Here's how the part is built. I have some questions about the finished solid (model axes, mm). Coordinates: 2 decimals unless noted, no trailing zeros. Loops run counter-clockwise (first coordinate to the right, second up) from the corner with the lowest first, then second, coordinate; pieces in that order, holes last. Notation, with made-up numbers: (-40, -12.75) -> (19, -12.75) arc R9 ccw to (19, -1.75) -> close; hole circle Ø6 at (23.5, -35.75). An arc over 180 degrees is marked (long way). Answer as a JSON object with one key per item and string values. Group by question number.
1) I want a section at B-B (z = 1.7). Write out the boundary of the cut face in (x, y), then the cut area to 3 significant figures.
2) I want a section at D-D (y = 14). Write out the boundary of the cut face in (x, z).
3) If we mould it in two halves opening along X, with no side actions, what happens to faces 1 (the cylindrical face through (-1.08, -4.88, 1.52)), 2 (the cylindrical face through (-195.23, 1.5, 1.52)), 3 (the flat face through (-98, 0, 0)), 4 (the cylindrical face through (-216, 0, 1))? For each: +X half, -X half, draft (parallel to the pull), parting line (faces both ways), or undercut.
4) I need wall thicknesses on probe 1 along X at (y, z) = (-1, 2.85); probe 2 along X at (y, z) = (2, 0.1); probe 3 along Y at (x, z) = (-2, 1.25). Which ranges of each line are inside material? Lowest first, please. Write a range as [from, to].
5) I want a section at C-C (y = -13). Write out the boundary of the cut face in (x, z), then the cut area to 3 significant figures.
6) I want a section at A-A (y = 0). Write out the boundary of the cut face in (x, z), then the cut area to 3 significant figures.
```python
from build123d import *

# Parameters (mm, degrees)
EXTRUDE_1_DEPTH     = 3
SKETCH_2_R          = 5
CUT_EXTRUDE_1_DEPTH = 3


with BuildPart() as part:
    # 草图1 → 凸台-拉伸1 (new body)
    with BuildSketch(Plane.XY):
        with BuildLine():
            Line((0, -16), (-200, -16))
            ThreePointArc((-200, -16), (-216, 0), (-200, 16))
            Line((-200, 16), (0, 16))
            ThreePointArc((0, 16), (16, 0), (0, -16))
        make_face()
    extrude(amount=EXTRUDE_1_DEPTH)

    # 草图2 → 切除-拉伸1 (cut)
    with BuildSketch(Plane.XY.offset(3)):
        with Locations((-200, 0)):
            Circle(SKETCH_2_R)
        Circle(SKETCH_2_R)
    extrude(amount=-CUT_EXTRUDE_1_DEPTH, mode=Mode.SUBTRACT)


solid = part.part
```
Determined:
{
 "1": {"outline": "(-200, -16) -> (0, -16) arc R16 ccw to (0, 16) -> (-200, 16) arc R16 ccw to start; hole circle Ø10 at (-200, 0); hole circle Ø10 at (0, 0)", "area": "7,050 mm^2"},
 "2": {"outline": "(-207.75, 0) -> (7.75, 0) -> (7.75, 3) -> (-207.75, 3) -> close"},
 "3": {"face 1": "undercut", "face 2": "undercut", "face 3": "draft", "face 4": "-X half"},
 "4": {"probe 1": "[-215.97, -204.9], [-195.1, -4.9], [4.9, 15.97]", "probe 2": "[-215.87, -204.58], [-195.42, -4.58], [4.58, 15.87]", "probe 3": "[-16, -4.58], [4.58, 16]"},
 "5": {"outline": "(-209.33, 0) -> (9.33, 0) -> (9.33, 3) -> (-209.33, 3) -> close", "area": "656 mm^2"},
 "6": {"outline": "(-216, 0) -> (-205, 0) -> (-205, 3) -> (-216, 3) -> close; (-195, 0) -> (-5, 0) -> (-5, 3) -> (-195, 3) -> close; (5, 0) -> (16, 0) -> (16, 3) -> (5, 3) -> close", "area": "636 mm^2"}
}
